For this review, take the finished solid that the model builds, in its own axes (mm). A direction names the side the tool comes from. Give positions to 0.01 mm unless a question says otherwise; leave off trailing zeros. Order: outer loops, then holes, each group sorted by start corner. A loop starts at its lowest first (then second) coordinate and runs counter-clockwise, first axis right, second up. Notation, with made-up numbers: (85.25, -13.75) - (138.25, -13.75) arc R22 ccw to (138.25, -2.75) - close; hole circle Ø6 at (39.25, -22). An arc over 180 degrees is marked (long way). One line per item, written item: value.
```python
from build123d import *

# Parameters (mm, degrees)
SKETCH2_R          = 1
CUT_EXTRUDE1_DEPTH = 1


with BuildPart() as part:
    # Sketch1 → Revolve1 (revolve)
    with BuildSketch(Plane.XY, mode=Mode.PRIVATE) as revolve1_sk:
        Polygon((0, 19), (1, 19), (1, 16.5), (2, 16.5), (2, 17), (4, 17), (4, 15), (1.5, 15), (1.5, 0), (0, 0), align=None)
    revolve(revolve1_sk.sketch.rotate(Axis((0, 0, 0), (1, 0, 0)), 90), axis=Axis((0, 0, 0), (1, 0, 0)))

    # Sketch2 → Cut-Extrude1 (cut)
    with BuildSketch(Plane.ZY):
        with Locations((-10, 0)):
            Circle(SKETCH2_R)
        with Locations((0, 10)):
            Circle(SKETCH2_R)
        with Locations((10, 0)):
            Circle(SKETCH2_R)
        with Locations((0, -10)):
            Circle(SKETCH2_R)
    extrude(amount=-CUT_EXTRUDE1_DEPTH, mode=Mode.SUBTRACT)


solid = part.part
```
(1) Machinability: for faces 1 (the face through (1, 10, 0)), 2 (the face through (4, 14, 6)), 3 (the face through (2.73, -12.65, 8.06)), 4 (the face through (1, -16, -6)), which of the approach directions +Z, -Z, +X, -X, +Y, -Y give a long, thin tool a straight path to every point of the face, cutting with its end or side? Answer none if there is none.
Answers below:
face 1: -X
face 2: +Z, -Z, +X, +Y, -Y
face 3: +X
face 4: none
(2) Wall thickness on line 1 (Y direction, x = 0.4, z = 0); line 2 (X direction, y = -16, z = -5.5); line 3 (X direction, y = -16.5, z = 7): over which ranges is each line inside the solid? List them lowest first. Write a range as from..to.
Answers below:
line 1: y = -19..-11, -9..9, 11..19
line 2: x = 0..1, 2..4
line 3: x = 0..1
(3) Take a section at A-A (y = 0). Write out the cut boundary in (x, z).
Answers below:
outline: (0, -19) - (1, -19) - (1, -16.5) - (2, -16.5) - (2, -17) - (4, -17) - (4, -15) - (1.5, -15) - (1.5, 15) - (4, 15) - (4, 17) - (2, 17) - (2, 16.5) - (1, 16.5) - (1, 19) - (0, 19) - (0, 11) - (1, 11) - (1, 9) - (0, 9) - (0, -9) - (1, -9) - (1, -11) - (0, -11) - close
(4) Draft analysis for pull direction X (two halves, no side actions). For faces 5 (the face through (2, -2.6, 16.45)), 6 (the face through (3.014, -16.855, -2.213)), 7 (the face through (1.5, 0, 0)), 8 (the face through (1.507, -4.956, 15.738)), state which applies: pulls with the +X half, pulls with the -X half, needs draft (parallel to the pull), parting line crosses it, or undercut.
Answers below:
face 5: undercut
face 6: needs draft
face 7: pulls with the +X half
face 8: undercut
(5) Take a section at D-D (x = 3). Write out the cut boundary in (y, z), then the cut area to 3 significant figures.
Answers below:
outline: circle Ø34 at (0, 0); hole circle Ø30 at (0, 0)
area: 201 mm^2
(6) Take a section at C-C (x = 0.5). Write out the cut boundary in (y, z), then the cut area to 3 significant figures.
Answers below:
outline: circle Ø38 at (0, 0); hole circle Ø2 at (-10, 0); hole circle Ø2 at (0, -10); hole circle Ø2 at (0, 10); hole circle Ø2 at (10, 0)
area: 1,120 mm^2
(7) For P1, Ø11.5, axis at y = 3.5, z = 5.5, coming from the +X side; P2, Ø2, axis at x = 3.5, y = 5, coming from the -Z side; P3, Ø1.6, axis at y = 0, z = 10, coming from the -X side, all flat-tipped, find the tip position at first contact; note any pin that passes through.
Answers below:
P1: stops at x = 1.5
P2: stops at z = -16.52
P3: stops at x = 1
